```python
from build123d import *

# Parameters (mm, degrees)
SKETCH1_W           = 40
SKETCH1_H           = 40
BOSS_EXTRUDE1_DEPTH = 40
CUT_EXTRUDE1_DEPTH  = 40
CUT_EXTRUDE2_DEPTH  = 40


with BuildPart() as part:
    # Sketch1 → Boss-Extrude1 (new body)
    with BuildSketch(Plane.XY):
        with Locations((20, 20)):
            Rectangle(SKETCH1_W, SKETCH1_H)
    extrude(amount=BOSS_EXTRUDE1_DEPTH)

    # Sketch2 → Cut-Extrude1 (cut)
    with BuildSketch(Plane.ZY):
        Polygon((20, 40), (40, 20), (40, 40), align=None)
        Polygon((40, 20), (20, 0), (40, 0), align=None)
    extrude(amount=-CUT_EXTRUDE1_DEPTH, mode=Mode.SUBTRACT)

    # Sketch3 → Cut-Extrude2 (cut)
    with BuildSketch(Plane(origin=(0, 0, 0), x_dir=(0, 0, -1), z_dir=(1, 0, 0))):
        Polygon((-20, 40), (0, 20), (0, 40), align=None)
    extrude(amount=CUT_EXTRUDE2_DEPTH, mode=Mode.SUBTRACT)


solid = part.part
```
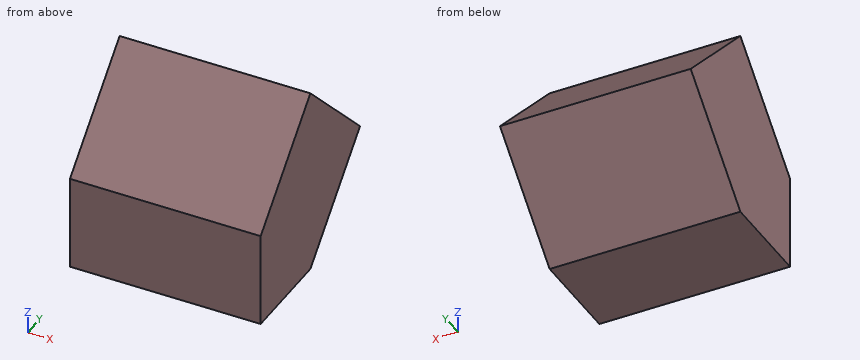
Geometry check sheet. Reference: the model listing, model coordinates, mm. Give positions to 0.01 mm unless a question says otherwise; leave off trailing zeros. Order: outer loops, then holes, each group sorted by start corner. A loop starts at its lowest first (then second) coordinate and runs counter-clockwise, first axis right, second up. Notation, with made-up numbers: (18, 25.25) -> (51, 25.25) arc R10 cw to (51, 43.25) -> close; hole circle Ø10 at (78, 74). An arc over 180 degrees is marked (long way). Write each question's results on one line, items separated by ' | '. Start each with the question number.
(1) Sectioned sample at A-A (x = 17.5). Enter the section's corners in (y, z), plus the area to 3 significant figures.
(2) Scan lines: line 1 (Y direction, x = 37, z = 24); line 2 (Y direction, x = 29, z = 38.5); line 3 (Z direction, x = 38, y = 8). Record each from-to range of solid material in increasing order.
(3) Gauge pin test, flat ends, axial feed: P1, Ø10, axis at x = 28, z = 9.5, coming from the -Y side; P2, Ø10, axis at x = 4.5, z = 8, coming from the +Y side; P3, Ø2, axis at x = 25.5, y = 26, coming from the -Z side; P4, Ø8, axis at x = 19, z = 26, coming from the -Y side. Record the tip position at first contact, or that the pin passes through.
(4) Sectioned sample at B-B (z = 29.5). Enter the section's corners in (x, y), plus the area to 3 significant figures.
(5) Sectioned sample at C-C (y = 13). Enter the section's corners in (x, z).
Answer below:
1) outline: (0, 0) -> (20, 0) -> (40, 20) -> (20, 40) -> (0, 20) -> close | area: 1,000 mm2
2) line 1: 4 to 36 | line 2: 18.5 to 21.5 | line 3: 0 to 28
3) P1: y = 0 | P2: y = 33 | P3: z = 5 | P4: y = 2
4) outline: (0, 9.5) -> (40, 9.5) -> (40, 30.5) -> (0, 30.5) -> close | area: 840 mm2
5) outline: (0, 0) -> (40, 0) -> (40, 33) -> (0, 33) -> close
